Geometry check sheet. Reference: drawing and pictorial views, mm from the part's lowest x, y, z. A direction names the side the tool comes from. Coordinates: 2 decimals unless noted, no trailing zeros. Loops run counter-clockwise (first coordinate to the right, second up) from the corner with the lowest first, then second, coordinate; pieces in that order, holes last. Notation, with made-up numbers: (9.25, 35) -> (19.25, 35) arc R21 ccw to (19.25, 40) -> close; hole circle Ø2 at (67.25, 63.25). An arc over 180 degrees is marked (long way). Answer as a JSON object with one key per item and string values. Group by question number.
Q1. Cross-section at D-D on z = 12.7. Record the boundary of the cut face in (x, y) (1 decimal).
Q2. Cross-section at B-B on x = 6.35. Record the boundary of the cut face in (y, z) (1 decimal), and give its area (3 significant figures).
Q3. Cross-section at C-C on y = 12.7. Record the boundary of the cut face in (x, z) (1 decimal).
Q4. Scan lines: L1, parallel to X at y = 0.7, z = 12.7; L2, parallel to Z at x = 38.1, y = 2.05; L3, parallel to Y at x = 45, z = 3.75 (1 decimal). Record each from-to range of solid material in increasing order.
Q5. Release check for a two-part mould opening along Y. For the marked faces 1, 2, 3 and 4 record: released by +Y, released by -Y, zero draft, split by the parting line, or undercut.
Q6. Cross-section at A-A on x = 25.4. Record the boundary of the cut face in (y, z) (1 decimal).
Q7. Gauge pin test, flat ends, axial feed: pin 1 Ø11 at (x, y) = (29, 9) entering from +Z (3 decimals); pin 2 Ø8.5 at (x, z) = (25.4, 12.7) entering from +Y (3 decimals). Record the tip position at first contact, or that the pin passes through.
Q8. Set-up check for the marked faces 5 and 6: record each of +Z, -Z, +X, -X, +Y, -Y from which the full face is reachable in a straight line by a thin tool's end or side.
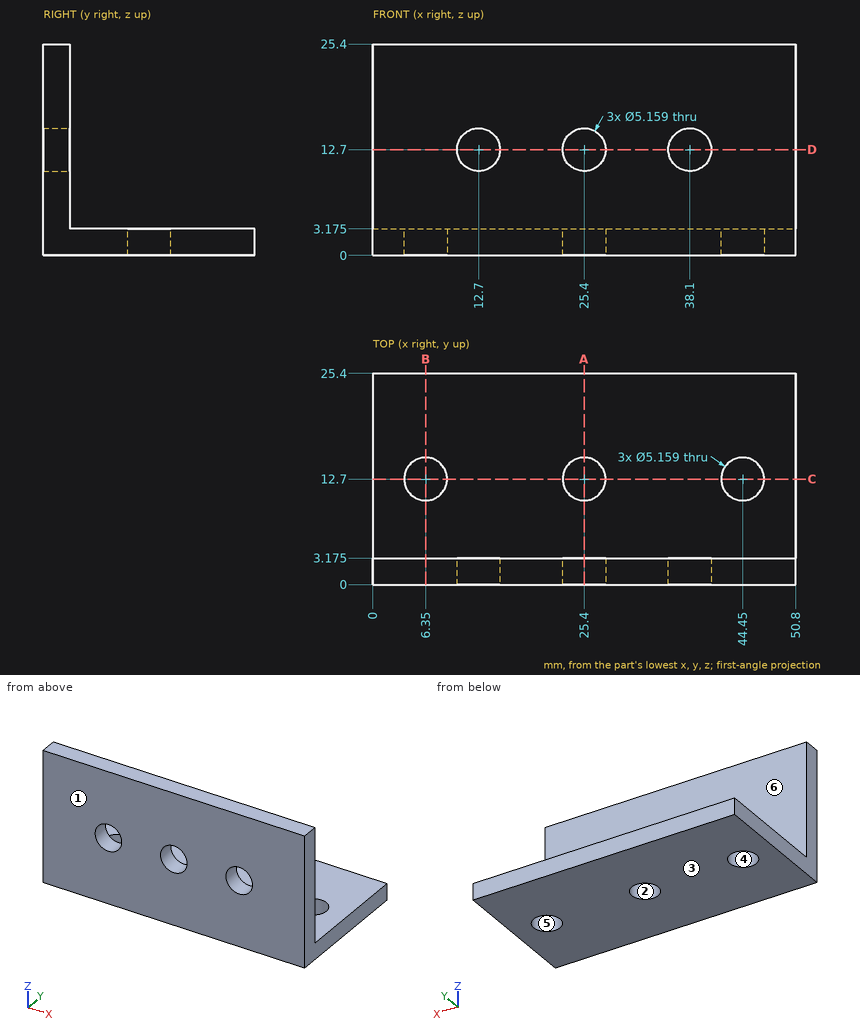
Computed values:
{
 "1": {"outline": "(0, 0) -> (10.1, 0) -> (10.1, 3.2) -> (0, 3.2) -> close; (15.3, 0) -> (22.8, 0) -> (22.8, 3.2) -> (15.3, 3.2) -> close; (28, 0) -> (35.5, 0) -> (35.5, 3.2) -> (28, 3.2) -> close; (40.7, 0) -> (50.8, 0) -> (50.8, 3.2) -> (40.7, 3.2) -> close"},
 "2": {"outline": "(0, 0) -> (10.1, 0) -> (10.1, 3.2) -> (3.2, 3.2) -> (3.2, 25.4) -> (0, 25.4) -> close; (15.3, 0) -> (25.4, 0) -> (25.4, 3.2) -> (15.3, 3.2) -> close", "area": "135 mm²"},
 "3": {"outline": "(0, 0) -> (3.8, 0) -> (3.8, 3.2) -> (0, 3.2) -> close; (8.9, 0) -> (22.8, 0) -> (22.8, 3.2) -> (8.9, 3.2) -> close; (28, 0) -> (41.9, 0) -> (41.9, 3.2) -> (28, 3.2) -> close; (47, 0) -> (50.8, 0) -> (50.8, 3.2) -> (47, 3.2) -> close"},
 "4": {"L1": "x = 0 to 10.12, 15.28 to 22.82, 27.98 to 35.52, 40.68 to 50.8", "L2": "z = 0 to 10.12, 15.28 to 25.4", "L3": "y = 0 to 3.2"},
 "5": {"face 1": "released by -Y", "face 2": "undercut", "face 3": "zero draft", "face 4": "undercut"},
 "6": {"outline": "(0, 0) -> (10.1, 0) -> (10.1, 3.2) -> (3.2, 3.2) -> (3.2, 10.1) -> (0, 10.1) -> close; (0, 15.3) -> (3.2, 15.3) -> (3.2, 25.4) -> (0, 25.4) -> close; (15.3, 0) -> (25.4, 0) -> (25.4, 3.2) -> (15.3, 3.2) -> close"},
 "7": {"pin 1": "stops at z = 3.175", "pin 2": "stops at y = 3.175"},
 "8": {"face 5": "+Z, -Z", "face 6": "+Z, +X, -X, +Y"}
}
